Design review of the part built by this model. Coordinates are the model's own, in mm. Face numbers are marked on the shaded views. Round coordinates to 2 decimals unless told otherwise and drop trailing zeros. Loops run counter-clockwise (first coordinate to the right, second up) from the corner with the lowest first, then second, coordinate; pieces in that order, holes last. Notation, with made-up numbers: (56.25, 63) - (73.25, 63) arc R20 cw to (73.25, 70) - close; hole circle Ø11 at (-5, 78). An arc over 180 degrees is marked (long way). Return JSON: item names as keys, results as strings. Group by question number.
(1) We need section D-D, the plane x = 3.25. Write out the cut boundary in (y, z).
(2) Clearance check with flat-ended pins moving along their axes: pin 1 (12 mm diameter, centred on x = 3.5, z = 6, fed in from -Y); pin 2 (5 mm diameter, centred on x = 4, z = 12.5, fed in from -Y); pin 3 (8 mm diameter, centred on y = 7, z = 7.5, fed in from +X); pin 4 (0.5 mm diameter, centred on x = 2, y = 0.5, fed in from -Z). State where each tip first meets the part, or that it passes through.
(3) We need section B-B, the plane z = 1.75. Write out the cut boundary in (x, y), and give its area (3 significant figures).
(4) The part is to be moulded in two halves that separate along X. For the marked faces 1, 2 and 3, say which applies: pulls with the +X half, pulls with the -X half, needs draft (parallel to the pull), parting line crosses it, or undercut.
(5) We need section C-C, the plane z = 14.25. Write out the cut boundary in (x, y) (3 decimals).
(6) We need section A-A, the plane x = 0. Write out the cut boundary in (y, z) (3 decimals), and give its area (3 significant figures).
(7) Wall thickness on L1, parallel to Z at x = -7.75, y = 1.25; L2, parallel to Y at x = 1, z = 12; L3, parallel to Y at x = -6.5, z = 4.25: over which ranges is each line inside the solid? List them lowest first. Write a range as [from, to].
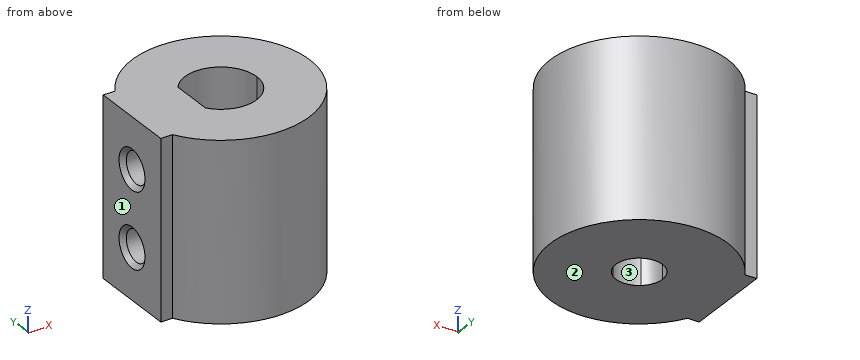
from build123d import *

# Parameters (mm, degrees)
SKETCH1_R                = 10.05
BOSS_EXTRUDE1_DEPTH      = 20
CUT_EXTRUDE2_DEPTH       = 8.5
CUT_EXTRUDE3_DEPTH       = 3
CUT_EXTRUDE1_DEPTH       = 11.5
BOSS_EXTRUDE2_REACH      = 32.083
BOSS_EXTRUDE2_END_RADIUS = 10.05
SKETCH8_W                = 20
SKETCH8_H                = 10
SKETCH6_R                = 1.75
CUT_EXTRUDE4_DEPTH       = 8.45
CUT_EXTRUDE5_REACH       = 32.083
CHAMFER1_SIZE            = 0.5


with BuildPart() as part:
    # Sketch1 → Boss-Extrude1 (new body)
    with BuildSketch(Plane.XY):
        Circle(SKETCH1_R)
    extrude(amount=BOSS_EXTRUDE1_DEPTH)

    # Sketch4 → Cut-Extrude2 (cut)
    with BuildSketch(Plane(origin=(0, 0, 0), x_dir=(-1, 0, 0), z_dir=(0, 0, -1))):
        with BuildLine():
            Line((-1.6, -2.1), (-1.6, 2.1))
            ThreePointArc((-1.6, 2.1), (0, 2.625143683), (1.6, 2.1))
            Line((1.6, 2.1), (1.6, -2.1))
            ThreePointArc((1.6, -2.1), (0, -2.625143683), (-1.6, -2.1))
        make_face()
    extrude(amount=-CUT_EXTRUDE2_DEPTH, mode=Mode.SUBTRACT)

    # Sketch5 → Cut-Extrude3 (cut)
    with BuildSketch(Plane(origin=(0, 0, 0), x_dir=(-1, 0, 0), z_dir=(0, 0, -1))):
        with BuildLine():
            Line((-1.6, -2.1), (-1.6, 2.1))
            ThreePointArc((-1.6, 2.1), (-2.640075756, 0), (-1.6, -2.1))
        make_face()
        with BuildLine():
            ThreePointArc((1.6, -2.1), (2.365810771, -1.171724966), (2.640075756, 0))
            ThreePointArc((2.640075756, 0), (2.365810771, 1.171724966), (1.6, 2.1))
            Line((1.6, 2.1), (1.6, -2.1))
        make_face()
    extrude(amount=-CUT_EXTRUDE3_DEPTH, mode=Mode.SUBTRACT)

    # Sketch3 → Cut-Extrude1 (cut)
    with BuildSketch(Plane.XY.offset(20)):
        with BuildLine():
            ThreePointArc((4.075, 0), (1.256607536, 3.876411033), (-3.3, 2.390737334))
            Line((-3.3, 2.390737334), (-3.3, -2.390737334))
            ThreePointArc((-3.3, -2.390737334), (1.256607536, -3.876411033), (4.075, 0))
        make_face()
    extrude(amount=-CUT_EXTRUDE1_DEPTH, mode=Mode.SUBTRACT)

    # Boss-Extrude2: up to this cylinder (the profile starts outside it)
    boss_extrude2_end = Plane(origin=(0, 0, 10), z_dir=(0, 0, -1)) * Cylinder(BOSS_EXTRUDE2_END_RADIUS, 85.266, mode=Mode.PRIVATE)
    # Sketch8 → Boss-Extrude2 (add, up to the surface)
    with BuildSketch(Plane.ZY.offset(10.05), mode=Mode.PRIVATE) as boss_extrude2_sk1:
        with Locations((10, 0)):
            Rectangle(SKETCH8_W, SKETCH8_H)
    boss_extrude2_tool1 = extrude(boss_extrude2_sk1.sketch, amount=-BOSS_EXTRUDE2_REACH, mode=Mode.PRIVATE) - boss_extrude2_end
    add(boss_extrude2_tool1.solids().sort_by_distance((-10.05, 0, 10))[0])
    add(boss_extrude2_tool1.solids().sort_by_distance((-10.05, 0, 10))[1])

    # Sketch6 → Cut-Extrude4 (cut)
    with BuildSketch(Plane.ZY.offset(10.05)):
        with Locations((5.75, 0)):
            Circle(SKETCH6_R)
    extrude(amount=-CUT_EXTRUDE4_DEPTH, mode=Mode.SUBTRACT)

    # Sketch7 → Cut-Extrude5 (cut, up to next)
    with BuildSketch(Plane.ZY.offset(10.05), mode=Mode.PRIVATE) as cut_extrude5_sk1:
        with BuildLine():
            ThreePointArc((16, 0), (14.25, 1.75), (12.5, 0))
            Line((12.5, 0), (16, 0))
        make_face()
    cut_extrude5_tool1 = extrude(cut_extrude5_sk1.sketch, amount=-CUT_EXTRUDE5_REACH, mode=Mode.PRIVATE) & part.part
    # Sketch7 → Cut-Extrude5 (cut, up to next)
    with BuildSketch(Plane.ZY.offset(10.05), mode=Mode.PRIVATE) as cut_extrude5_sk2:
        with BuildLine():
            Line((16, 0), (12.5, 0))
            ThreePointArc((12.5, 0), (14.25, -1.75), (16, 0))
        make_face()
    cut_extrude5_tool2 = extrude(cut_extrude5_sk2.sketch, amount=-CUT_EXTRUDE5_REACH, mode=Mode.PRIVATE) & part.part
    # Sketch7 → Cut-Extrude5 (cut, up to next)
    with BuildSketch(Plane.ZY.offset(10.05), mode=Mode.PRIVATE) as cut_extrude5_sk3:
        with BuildLine():
            ThreePointArc((16, 0), (14.25, 1.75), (12.5, 0))
            Line((12.5, 0), (16, 0))
        make_face()
    cut_extrude5_tool3 = extrude(cut_extrude5_sk3.sketch, amount=-CUT_EXTRUDE5_REACH, mode=Mode.PRIVATE) & part.part
    # Sketch7 → Cut-Extrude5 (cut, up to next)
    with BuildSketch(Plane.ZY.offset(10.05), mode=Mode.PRIVATE) as cut_extrude5_sk4:
        with BuildLine():
            Line((16, 0), (12.5, 0))
            ThreePointArc((12.5, 0), (14.25, -1.75), (16, 0))
        make_face()
    cut_extrude5_tool4 = extrude(cut_extrude5_sk4.sketch, amount=-CUT_EXTRUDE5_REACH, mode=Mode.PRIVATE) & part.part
    add(cut_extrude5_tool1.solids().sort_by_distance((-10.05, 0.742723, 14.25))[0], mode=Mode.SUBTRACT)
    add(cut_extrude5_tool2.solids().sort_by_distance((-10.05, -0.742723, 14.25))[0], mode=Mode.SUBTRACT)
    add(cut_extrude5_tool3.solids().sort_by_distance((-10.05, 0.742723, 14.25))[0], mode=Mode.SUBTRACT)
    add(cut_extrude5_tool4.solids().sort_by_distance((-10.05, -0.742723, 14.25))[0], mode=Mode.SUBTRACT)

    # Chamfer1
    chamfer1_edges = [part.edges().sort_by_distance(p)[0] for p in [
        (-10.05, 0, 4),
        (-10.05, 0, 12.5),
    ]]
    chamfer(chamfer1_edges, length=CHAMFER1_SIZE)


solid = part.part
Solutions:
{
 "1": {"outline": "(-9.51, 0) - (9.51, 0) - (9.51, 20) - (2.46, 20) - (2.46, 8.5) - (-2.46, 8.5) - (-2.46, 20) - (-9.51, 20) - close"},
 "2": {"pin 1": "y = -10.05", "pin 2": "y = -9.94", "pin 3": "x = 9.59", "pin 4": "z = 3"},
 "3": {"outline": "(-10.05, -5) - (-8.72, -5) arc R10.05 ccw (long way) to (-8.72, 5) - (-10.05, 5) - close; hole (-1.6, -2.1) arc R2.7 ccw to (1.6, -2.1) arc R2.64 ccw to (1.6, 2.1) arc R2.7 ccw to (-1.6, 2.1) arc R2.64 ccw to start", "area": "300 mm^2"},
 "4": {"face 1": "pulls with the -X half", "face 2": "needs draft", "face 3": "undercut"},
 "5": {"outline": "(-10.05, -5) - (-8.718, -5) arc R10.05 ccw (long way) to (-8.718, 5) - (-10.05, 5) - (-10.05, 2.25) - (-9.55, 1.75) - (-3.3, 1.75) - (-3.3, 2.391) arc R4.075 cw (long way) to (-3.3, -2.391) - (-3.3, -1.75) - (-9.55, -1.75) - (-10.05, -2.25) - close"},
 "6": {"outline": "(-10.05, 0) - (-2.625, 0) - (-2.625, 8.5) - (-4.075, 8.5) - (-4.075, 20) - (-10.05, 20) - close; (2.625, 0) - (10.05, 0) - (10.05, 20) - (4.075, 20) - (4.075, 8.5) - (2.625, 8.5) - close", "area": "264 mm^2"},
 "7": {"L1": "[0, 4.53], [6.97, 13.03], [15.47, 20]", "L2": "[-10, -3.95], [3.95, 10]", "L3": "[-7.67, -0.9], [0.9, 7.67]"}
}
